Source: CAD feature listing. Evaluate the final solid. Frame: model axes, mm. A direction names the side the tool comes from. Give positions to 0.01 mm unless a question says otherwise; leave off trailing zeros. Loops run counter-clockwise (first coordinate to the right, second up) from the corner with the lowest first, then second, coordinate; pieces in that order, holes last. Notation, with made-up numbers: (40, 60.5) - (84, 60.5) arc R11 ccw to (84, 71.5) - close; hole circle Ø10 at (86, 17.25). An arc over 180 degrees is marked (long way). Put each result on its own line as item: value.
```python
from build123d import *

# Parameters (mm, degrees)
SKETCH_1_W          = 12
SKETCH_1_H          = 10
EXTRUDE_1_DEPTH     = 24
FILLET_1_R          = 1
CUT_EXTRUDE_START   = -15.1
SKETCH_2_OUTSIDE_W  = 19.728
SKETCH_2_OUTSIDE_H  = 17.728
CUT_EXTRUDE_1_DEPTH = 15.1
SKETCH_3_R          = 1.5
EXTRUDE_2_DEPTH     = 14
SKETCH_5_R          = 2.5
EXTRUDE_3_DEPTH     = 1.25
SKETCH_6_W          = 20
SKETCH_6_H          = 4.3
SKETCH_6_H_2        = 2.29
CUT_EXTRUDE_2_REACH = 28.43
SKETCH_4_R          = 0.8
EXTRUDE_START       = -8.13
EXTRUDE_4_DEPTH     = 7.36


with BuildPart() as part:
    # 草图1 → 凸台-拉伸1 (new body)
    with BuildSketch(Plane(origin=(0, 0, 0), x_dir=(1, 0, 0), z_dir=(0, 1, 0))):
        Rectangle(SKETCH_1_W, SKETCH_1_H)
    extrude(amount=EXTRUDE_1_DEPTH)

    # 圆角1
    fillet_1_edges = [part.edges().sort_by_distance(p)[0] for p in [
        (6, 12, 5),
        (-6, 12, 5),
        (-6, 12, -5),
        (6, 12, -5),
    ]]
    fillet(fillet_1_edges, radius=FILLET_1_R)

    # 草图2 outside → 切除-拉伸1 (cut)
    with BuildSketch(Plane.XZ.offset(CUT_EXTRUDE_START)):
        Rectangle(SKETCH_2_OUTSIDE_W, SKETCH_2_OUTSIDE_H)
        with BuildLine():
            Line((-3.31662479, -5), (3.31662479, -5))
            ThreePointArc((3.31662479, -5), (5.286764074, -2.837274331), (6, 0))
            ThreePointArc((6, 0), (5.286764074, 2.837274331), (3.31662479, 5))
            Line((3.31662479, 5), (-3.31662479, 5))
            ThreePointArc((-3.31662479, 5), (-5.286764074, 2.837274331), (-6, 0))
            ThreePointArc((-6, 0), (-5.286764074, -2.837274331), (-3.31662479, -5))
        make_face(mode=Mode.SUBTRACT)
    extrude(amount=CUT_EXTRUDE_1_DEPTH, mode=Mode.SUBTRACT)

    # 草图3 → 凸台-拉伸2 (add)
    with BuildSketch(Plane(origin=(0, 24, 0), x_dir=(1, 0, 0), z_dir=(0, 1, 0))):
        with Locations(Location((0, 0, 0), (0, 0, 270))):
            Circle(SKETCH_3_R)
    extrude(amount=EXTRUDE_2_DEPTH)

    # 草图5 → 凸台-拉伸3 (add)
    with BuildSketch(Plane.XZ):
        with Locations(Location((0, 0, 0), (0, 0, 270))):
            Circle(SKETCH_5_R)
    extrude(amount=EXTRUDE_3_DEPTH)

    # 草图6 → 切除-旋转3 (revolve, cut)
    with BuildSketch(Plane.XY, mode=Mode.PRIVATE) as cut_revolve_3_sk:
        with Locations((11.5, 21.08)):
            Rectangle(SKETCH_6_W, SKETCH_6_H)
        with Locations((11.5, 17.015)):
            Rectangle(SKETCH_6_W, SKETCH_6_H_2)
    revolve(cut_revolve_3_sk.sketch.rotate(Axis((0, 38, 0), (0, -1, 0)), 90), axis=Axis((0, 38, 0), (0, -1, 0)), mode=Mode.SUBTRACT)

    # 草图4 → 切除-拉伸2 (cut, up to next)
    with BuildSketch(Plane(origin=(0, 24, 0), x_dir=(1, 0, 0), z_dir=(0, 1, 0)), mode=Mode.PRIVATE) as cut_extrude_2_sk1:
        with Locations(Location((-4.5, 0, 0), (0, 0, 270))):
            Circle(SKETCH_4_R)
    cut_extrude_2_tool1 = extrude(cut_extrude_2_sk1.sketch, amount=-CUT_EXTRUDE_2_REACH, mode=Mode.PRIVATE) & part.part
    # 草图4 → 切除-拉伸2 (cut, up to next)
    with BuildSketch(Plane(origin=(0, 24, 0), x_dir=(1, 0, 0), z_dir=(0, 1, 0)), mode=Mode.PRIVATE) as cut_extrude_2_sk2:
        with Locations(Location((4.5, 0, 0), (0, 0, 270))):
            Circle(SKETCH_4_R)
    cut_extrude_2_tool2 = extrude(cut_extrude_2_sk2.sketch, amount=-CUT_EXTRUDE_2_REACH, mode=Mode.PRIVATE) & part.part
    add(cut_extrude_2_tool1.solids().sort_by_distance((-4.5, 24, 0))[0], mode=Mode.SUBTRACT)
    add(cut_extrude_2_tool2.solids().sort_by_distance((4.5, 24, 0))[0], mode=Mode.SUBTRACT)

    # 草图7 → 凸台-拉伸4 (add)
    with BuildSketch(Plane(origin=(0, 24, 0), x_dir=(1, 0, 0), z_dir=(0, 1, 0)).offset(EXTRUDE_START)):
        with BuildLine():
            ThreePointArc((3.75, 1.25), (4.810660172, 1.689339828), (5.25, 2.75))
            ThreePointArc((5.25, 2.75), (4.810660174, 3.81066017), (3.750000005, 4.25))
            ThreePointArc((3.750000005, 4.25), (2.68933983, 3.810660174), (2.25, 2.75))
            Line((2.25, 2.75), (3.75, 2.75))
            Line((3.75, 2.75), (3.75, 1.25))
        make_face()
        with BuildLine():
            ThreePointArc((2.25, 2.75), (2.689339828, 1.689339828), (3.75, 1.25))
            Line((3.75, 1.25), (3.75, 2.75))
            Line((3.75, 2.75), (2.25, 2.75))
        make_face()
        with BuildLine():
            ThreePointArc((-5.25, -2.750000006), (-4.810660171, -3.810660173), (-3.750000004, -4.25))
            ThreePointArc((-3.750000004, -4.25), (-2.68933983, -3.810660173), (-2.25, -2.75))
            Line((-2.25, -2.75), (-3.75, -2.75))
            Line((-3.75, -2.75), (-3.75, -1.25))
            ThreePointArc((-3.75, -1.25), (-4.810660174, -1.68933983), (-5.25, -2.750000006))
        make_face()
        with BuildLine():
            Line((-3.75, -2.75), (-2.25, -2.75))
            ThreePointArc((-2.25, -2.75), (-2.689339828, -1.689339828), (-3.75, -1.25))
            Line((-3.75, -1.25), (-3.75, -2.75))
        make_face()
    extrude(amount=EXTRUDE_4_DEPTH)


solid = part.part
```
1) Section query A-A, the plane y = 22. Output: boundary loops of the cut face in (x, z), plus the area to 3 significant figures.
Check result:
outline: circle Ø3 at (-3.75, 2.75); circle Ø3 at (0, 0); circle Ø3 at (3.75, -2.75)
area: 21.2 mm²
2) Material intervals for line 1 along Y through (x, z) = (-0.5, 1.5); line 2 along Y through (x, z) = (4.25, -1.25); line 3 along X through (y, z) = (23.85, 0), sorted ascending. Write a range as [from, to].
Check result:
line 1: [-1.25, 15.87], [18.16, 18.93], [23.23, 24]
line 2: [0, 15.87], [18.16, 18.93], [23.23, 24]
line 3: [-6, -5.3], [-3.7, 3.7], [5.3, 6]
3) Access query for faces 1 (the cylindrical face through (-2.44, -0.62, 0.54)), 2 (the cylindrical face through (-5.28, 23.62, -0.17)), 3 (the flat face through (-1.4, 23.23, -1)), 4 (the flat face through (5, 15.1, -4)). Directions: +Z, -Z, +X, -X, +Y, -Y. A direction counts if a zero-diameter tool reaches every point of the face in a straight line with its end or side. Return the directions, or none.
Check result:
face 1: -Y
face 2: +Y
face 3: none
face 4: -Z, +X, -Y
4) Section query C-C, the plane x = 4.5. Output: boundary loops of the cut face in (y, z), plus the area to 3 significant figures.
Check result:
outline: (0, -3.97) - (15.1, -3.97) - (15.1, -5) - (15.87, -5) - (15.87, -4.05) - (18.16, -4.05) - (18.16, -5) - (18.93, -5) - (18.93, -4.05) - (23.23, -4.05) - (23.23, -5) - (24, -5) - (24, -0.8) - (23.23, -0.8) - (23.23, -1.45) - (18.93, -1.45) - (18.93, 5) - (18.16, 5) - (18.16, -1.45) - (15.87, -1.45) - (15.87, 5) - (15.1, 5) - (15.1, 3.97) - (0, 3.97) - close; (23.23, 0.8) - (24, 0.8) - (24, 5) - (23.23, 5) - close
area: 159 mm²
5) Section query B-B, the plane x = 0. Output: boundary loops of the cut face in (y, z), plus the area to 3 significant figures.
Check result:
outline: (-1.25, -2.5) - (0, -2.5) - (0, -5) - (15.87, -5) - (15.87, -1.5) - (18.16, -1.5) - (18.16, -5) - (18.93, -5) - (18.93, -1.5) - (23.23, -1.5) - (23.23, -5) - (24, -5) - (24, -1.5) - (38, -1.5) - (38, 1.5) - (24, 1.5) - (24, 5) - (23.23, 5) - (23.23, 1.5) - (18.93, 1.5) - (18.93, 5) - (18.16, 5) - (18.16, 1.5) - (15.87, 1.5) - (15.87, 5) - (0, 5) - (0, 2.5) - (-1.25, 2.5) - close
area: 242 mm²
6) Mould query, pull axis Y, two halves, no side actions, for faces 5 (the flat face through (-1.4, 18.16, -1)), 6 (the flat face through (-1.4, 24, -1.2)), 7 (the cylindrical face through (-5.715, 18.55, -4.699)). Classes: pulls with the +Y half, pulls with the -Y half, needs draft (parallel to the pull), parting line crosses it, or undercut.
Check result:
face 5: undercut
face 6: pulls with the +Y half
face 7: needs draft
7) Pin query (flat end, axial travel): P1, Ø1, axis at x = -4, y = 10, coming from the -Z side; P2, Ø2, axis at x = -4.5, z = -3, coming from the -Y side; P3, Ø2, axis at x = -4.5, z = 0, coming from the +Y side. Return the tip coordinate at first contact, or that it passes through.
Check result:
P1: z = -4.87
P2: y = 0
P3: y = 24
